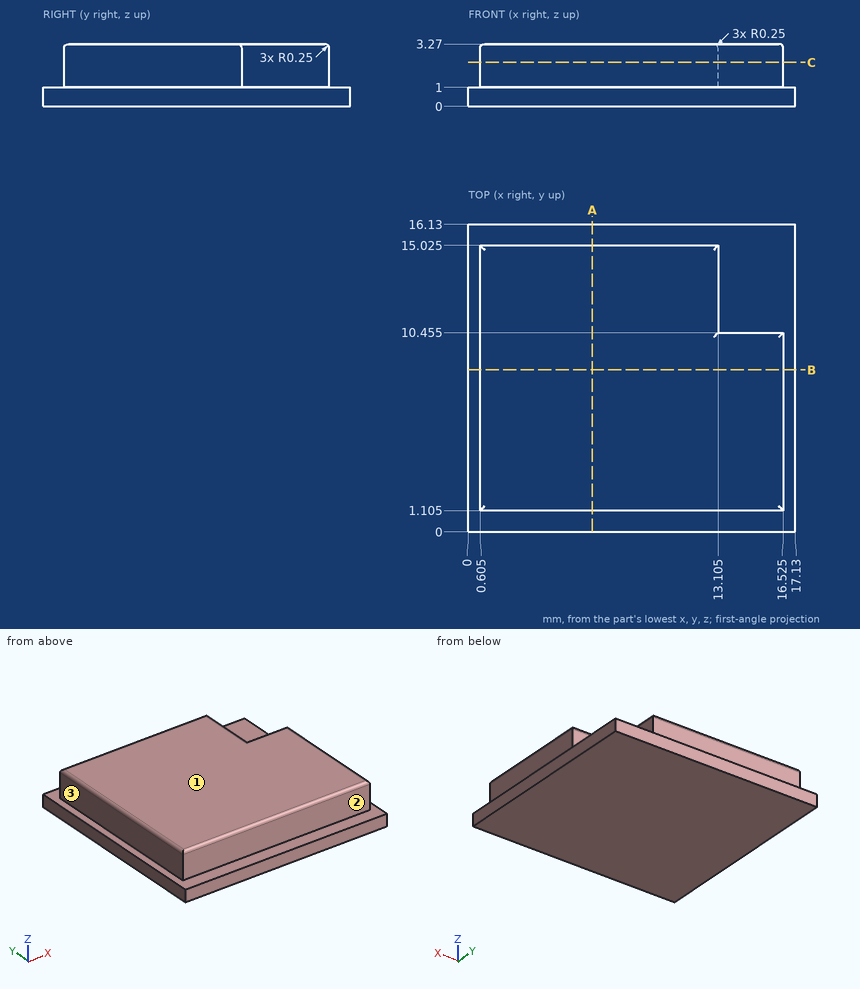
Part print with two shaded views. Sizes in mm from the minimum x, y, z corner. A direction names the side the tool comes from. Coordinates: 2 decimals unless noted, no trailing zeros. Loops run counter-clockwise (first coordinate to the right, second up) from the corner with the lowest first, then second, coordinate; pieces in that order, holes last. Notation, with made-up numbers: M 73.25,39.5 L 84.25,39.5 A27 ccw 84.25,56.5 Z; hole C -31,-11.5 d3. An arc over 180 degrees is marked long. Use CSV: the item, a comma, the result in double quotes. Start each with the question number.
1. Band-saw the part on C-C, the plane z = 2.3. List the corners of the cut face in (x, y) (3 decimals).
2. Probe probe 1 along Y at (x, z) = (12, 2.15) (3 decimals); probe 2 along X at (y, z) = (11, 2.35) (3 decimals); probe 3 along X at (y, z) = (5, 2.3) (3 decimals). List the from-to ranges inside material, lowest first. Write a range as [from, to].
3. Band-saw the part on B-B, the plane y = 8.5. List the corners of the cut face in (x, z) (3 decimals), then the cut area to 3 significant figures.
4. Flat gauge pins, fed straight in: pin 1 (1.6 mm diameter, centred on y = 6.5, z = 2, fed in from -X) (3 decimals); pin 2 (1.6 mm diameter, centred on y = 4, z = 2, fed in from +X) (3 decimals); pin 3 (1.6 mm diameter, centred on x = 14, z = 2, fed in from +Y) (3 decimals). Where does each tip first touch, or does it go through?
5. Band-saw the part on A-A, the plane x = 6.5. List the corners of the cut face in (y, z) (3 decimals).
6. Tool access for the marked faces 1, 2 and 3: list every direction of +Z, -Z, +X, -X, +Y, -Y with a clear straight run to the whole face (end or side of a thin tool).
Entries:
1,outline,"M 0.605,1.105 L 16.525,1.105 L 16.525,10.455 L 13.105,10.455 L 13.105,15.025 L 0.605,15.025 Z"
2,probe 1,"y = [1.105, 15.025]"
2,probe 2,"x = [0.605, 13.105]"
2,probe 3,"x = [0.605, 16.525]"
3,outline,"M 0,0 L 17.13,0 L 17.13,1 L 16.525,1 L 16.525,3.02 A0.25 ccw 16.275,3.27 L 0.855,3.27 A0.25 ccw 0.605,3.02 L 0.605,1 L 0,1 Z"
3,area,"53.2 mm2"
4,pin 1,"stops at x = 0.605"
4,pin 2,"stops at x = 16.525"
4,pin 3,"stops at y = 10.455"
5,outline,"M 0,0 L 16.13,0 L 16.13,1 L 15.025,1 L 15.025,3.02 A0.25 ccw 14.775,3.27 L 1.355,3.27 A0.25 ccw 1.105,3.02 L 1.105,1 L 0,1 Z"
6,face 1,"+Z, +X, -X, +Y, -Y"
6,face 2,"+Z, +X, -X, -Y"
6,face 3,"+Z, -X, +Y, -Y"
